Autodesk Inventor part; units mm, degrees
sketch "Эскиз1" plane through (0, 0, 0) normal (0, 0, 1) x (1, 0, 0)
  line L0 (-7, -15.75) -> (7, -15.75)
  line L1 (7, -15.75) -> (7, 15.75)
  line L2 (7, 15.75) -> (-7, 15.75)
  line L3 (-7, 15.75) -> (-7, -15.75)
  line L4 (-7, -15.75) -> (7, 15.75) construction
  line L5 (7, -15.75) -> (-7, 15.75) construction
  point P0 (0, 0)
  dimension "d0" = 14
  dimension "d1" = 31.5
extrude "Выдавливание1" add sketch "Эскиз1" along normal mid plane 5
sketch "Эскиз2" plane through (0, 0, -2.5) normal (0, 0, -1) x (-1, 0, 0)
  circle A0 centre (0, 8.75) radius 1.5
  circle A1 centre (0, 8.75) radius 2.5
  point P0 (0, 0)
  dimension "d7" = 1
sketch "Эскиз3" plane through (0, 0, -2.5) normal (0, 0, -1) x (-1, 0, 0)
  line L0 (-5.2, -14.88) -> (5.2, -14.88)
  line L1 (5.2, -14.88) -> (5.2, -8.98)
  line L2 (5.2, -8.98) -> (-5.2, -8.98)
  line L3 (-5.2, -8.98) -> (-5.2, -14.88)
  line L4 (-5.2, -14.88) -> (5.2, -8.98) construction
  line L5 (5.2, -14.88) -> (-5.2, -8.98) construction
  line L6 (-7, -15.75) -> (7, -15.75)
  line L7 (0, -22.05) -> (0, 22.05) construction
  point P0 (0, 0)
  point P1 (0, -11.93)
  dimension "d4" = 0.87
  dimension "d5" = 5.9
  dimension "d6" = 10.4
extrude "Выдавливание2" cut sketch "Эскиз2" against normal up to next contours A0 | A1
extrude "Выдавливание3" cut sketch "Эскиз3" against normal up to next
sketch "Эскиз4" plane through (0, 0, 2.5) normal (0, 0, 1) x (1, 0, 0)
  line L0 (-4.5, 13.75) -> (4.5, 13.75) construction
  line L1 (-4.5, 12.55) -> (4.5, 12.55)
  line L2 (4.5, 14.95) -> (-4.5, 14.95)
  arc A0 (-4.5, 14.95) -> (-4.5, 12.55) centre (-4.5, 13.75) ccw
  arc A1 (4.5, 12.55) -> (4.5, 14.95) centre (4.5, 13.75) ccw
  line L3 (7, 15.75) -> (-7, 15.75)
  line L4 (0, 22.05) -> (0, -22.05) construction
  point P0 (0, 0)
  point P1 (0, 13.75)
  dimension "d12" = 9
  dimension "d13" = 1.2
  dimension "d14" = 2
extrude "Выдавливание4" cut sketch "Эскиз4" against normal up to next
sketch "Эскиз5" plane through (0, 0, 2.5) normal (0, 0, 1) x (1, 0, 0)
  line L0 (-9.8, 0) -> (9.8, 0) construction
  line L1 (-5, 0) -> (5, 0) construction
  line L2 (5, 0) -> (5, -6.5)
  line L3 (5, -6.5) -> (-5, -6.5)
  line L4 (-5, -6.5) -> (-5, 0)
  line L5 (-5, 0) -> (5, 0) construction
  line L6 (5, 0) -> (5, 5)
  line L7 (5, 5) -> (-5, 5)
  line L8 (-5, 5) -> (-5, 0)
  line L9 (-5, 5) -> (5, -6.5) construction
  line L10 (5, 5) -> (-5, -6.5) construction
  line L11 (0, 22.05) -> (0, -22.05) construction
  point P0 (0, -0.75)
  dimension "d22" = 6.5
  dimension "d23" = 5
  dimension "d24" = 10
extrude "Выдавливание5" cut sketch "Эскиз5" against normal up to next
properties part number "Крепление_TCRT"
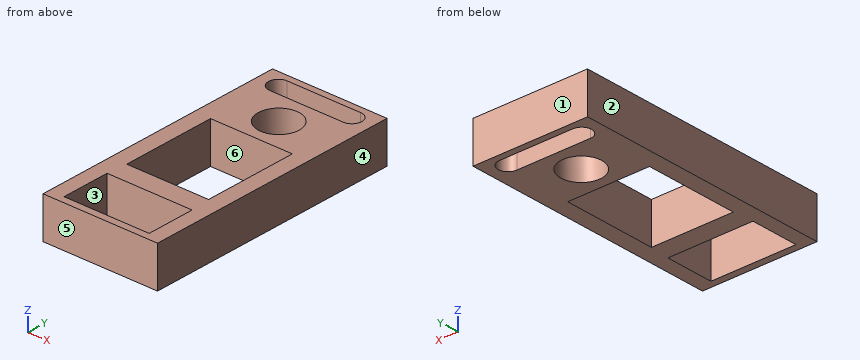
The model under review builds one solid part; all positions refer to its coordinate system, in mm. Face numbers are marked on the shaded views. A direction names the side the tool comes from. Give positions to 0.01 mm unless a question says otherwise; leave off trailing zeros. Write each loop counter-clockwise with the first axis right and the second up, starting at its lowest first coordinate (ties: lowest second). Pieces come first, ordered by that corner, then holes.
1. Add section A-A, the plane y = 13.75. Write out the cut boundary in (x, z), plus the area to 3 significant figures.
2. Add section B-B, the plane x = 0. Write out the cut boundary in (y, z).
3. Draft analysis for pull direction X (two halves, no side actions). For the marked faces 1, 2, 3 and 4, state which applies: +X half, -X half, draft (parallel to the pull), parting line (faces both ways), or undercut.
4. Add section D-D, the plane x = 3. Write out the cut boundary in (y, z), plus the area to 3 significant figures.
5. Tool access review of the marked faces 5 and 6: name each direction out of +Z, -Z, +X, -X, +Y, -Y from which nothing blocks a thin tool from reaching the whole face with its end or side.
6. Add section C-C, the plane z = -1.4. Write out the cut boundary in (x, y), plus the area to 3 significant figures.
7. Wall thickness on L1, parallel to Y at x = -4, z = -2.2; L2, parallel to Y at x = 0, z = -0.55; L3, parallel to X at y = 1, z = 1.15: over which ranges is each line inside the solid? List them lowest first.
Worked answers:
1. outline: (-7, -2.5) - (-5.7, -2.5) - (-5.7, 2.5) - (-7, 2.5) - close; (5.7, -2.5) - (7, -2.5) - (7, 2.5) - (5.7, 2.5) - close
1. area: 13.0 mm2
2. outline: (-15.75, -2.5) - (-14.88, -2.5) - (-14.88, 2.5) - (-15.75, 2.5) - close; (-8.98, -2.5) - (-6.5, -2.5) - (-6.5, 2.5) - (-8.98, 2.5) - close; (5, -2.5) - (6.25, -2.5) - (6.25, 2.5) - (5, 2.5) - close; (11.25, -2.5) - (12.55, -2.5) - (12.55, 2.5) - (11.25, 2.5) - close; (14.95, -2.5) - (15.75, -2.5) - (15.75, 2.5) - (14.95, 2.5) - close
3. face 1: draft
3. face 2: -X half
3. face 3: undercut
3. face 4: +X half
4. outline: (-15.75, -2.5) - (-14.88, -2.5) - (-14.88, 2.5) - (-15.75, 2.5) - close; (-8.98, -2.5) - (-6.5, -2.5) - (-6.5, 2.5) - (-8.98, 2.5) - close; (5, -2.5) - (12.55, -2.5) - (12.55, 2.5) - (5, 2.5) - close; (14.95, -2.5) - (15.75, -2.5) - (15.75, 2.5) - (14.95, 2.5) - close
4. area: 58.5 mm2
5. face 5: +Z, -Z, +X, -X, -Y
5. face 6: +Z, -Z
6. outline: (-7, -15.75) - (7, -15.75) - (7, 15.75) - (-7, 15.75) - close; hole (-5.2, -14.88) - (5.2, -14.88) - (5.2, -8.98) - (-5.2, -8.98) - close; hole (-5, -6.5) - (5, -6.5) - (5, 5) - (-5, 5) - close; hole (-4.5, 12.55) - (4.5, 12.55) arc R1.2 ccw to (4.5, 14.95) - (-4.5, 14.95) arc R1.2 ccw to start; hole circle Ø5 at (0, 8.75)
6. area: 219 mm2
7. L1: y = -15.75 to -14.88, -8.98 to -6.5, 5 to 12.55, 14.95 to 15.75
7. L2: y = -15.75 to -14.88, -8.98 to -6.5, 5 to 6.25, 11.25 to 12.55, 14.95 to 15.75
7. L3: x = -7 to -5, 5 to 7
